CAD build for the part. Positions are in the model's coordinates, mm. A direction names the side the tool comes from. Coordinates: 2 decimals unless noted, no trailing zeros. Order: outer loops, then holes, each group sorted by start corner. A loop starts at its lowest first (then second) coordinate and runs counter-clockwise, first axis right, second up. Notation, with made-up numbers: M 64,48.25 L 70,48.25 A30 ccw 70,83.25 Z; hole C 7,34 d10. An arc over 180 degrees is marked long. Write item = value, one per line.
from build123d import *

# Parameters (mm, degrees)
F1_R     = 1.99999
F2_DEPTH = 25
F6_R     = 2


# Not quite as in the source:
# - a fillet or chamfer that OpenCascade refuses, or shapes differently, is made with other operations: its cross-section is extruded or revolved along the edge and cut away or added
# - a fillet or chamfer is up to 0.001 mm smaller than in the source, because OpenCascade refuses the exact size


with BuildPart() as f0:
    # F3 (on Front) → F0 (revolve)
    with BuildSketch(Plane.XZ):
        Polygon((-2, 0), (0, 0), (0, 12), (-18.8, 12), (-18.8, 13.3), (-20.8, 13.3), (-20.8, 10.2), (-16.5, 10.2), (-15, 10.2), (-11.6, 10.2), (-10.1, 10.2), (-2, 10.2), align=None)
        Polygon((-14.9505181851, 9.7), (-15, 10.2), (-16.5, 10.2), align=None)
        Polygon((-10.2909830056, 9.7), (-10.1, 10.2), (-11.6, 10.2), align=None)
    revolve(axis=Axis((-1, 0, 0), (1, 0, 0)))

    # F1 (radius 2 in the source; OpenCascade refuses exactly that, so slightly less here)
    f1_edges = [f0.edges().sort_by_distance(p)[0] for p in [
        (-20.8, 0, -13.3),
    ]]
    fillet(f1_edges, radius=F1_R)

    # F4: fillet of radius 1.5 on 2 edges, made by hand

    # F4_s1 → F4_t2 (revolve, cut)
    with BuildSketch(Plane.XZ):
        with BuildLine():
            ThreePointArc((-16.1707444356, 10.0937530079), (-15.5745304293, 10.0274099354), (-15, 10.2))
            Line((-15, 10.2), (-14.9505181851, 9.7))
            Line((-14.9505181851, 9.7), (-16.1707444356, 10.0937530079))
        make_face()
    revolve(axis=Axis((-14.9505181851, 0, 0), (1, 0, 0)), mode=Mode.SUBTRACT)

    # F4_s3 → F4_t4 (revolve, cut)
    with BuildSketch(Plane.XZ):
        with BuildLine():
            ThreePointArc((-11.3639501712, 10.1098369884), (-10.721986782, 10.0148974609), (-10.1, 10.2))
            Line((-10.1, 10.2), (-10.2909830056, 9.7))
            Line((-10.2909830056, 9.7), (-11.3639501712, 10.1098369884))
        make_face()
    revolve(axis=Axis((-10.2909830056, 0, 0), (1, 0, 0)), mode=Mode.SUBTRACT)

    # F5 (on Top) → F2 (cut, symmetric)
    with BuildSketch(Plane.XY):
        Polygon((-7.8, 6.5), (-30.9797403524, 6.5), (-30.8855128417, -6.5), (-7.8, -6.5), align=None)
    extrude(amount=F2_DEPTH, both=True, mode=Mode.SUBTRACT)

    # F6
    f6_edges = [f0.edges().sort_by_distance(p)[0] for p in [
        (0, 0, -12),
    ]]
    fillet(f6_edges, radius=F6_R)


solid = f0.part
(1) Tool access for faces 1 (the face through (-18.8, -12.2, -0.8)), 2 (the face through (-16.333, -10.145, 0.125)), 3 (the face through (-13.3, -10.2, 0.1)), 4 (the face through (-18.8, 12.2, 0.1)), 5 (the face through (-7.8, -0.1, -10.4)): list every direction of +Z, -Z, +X, -X, +Y, -Y with a clear straight run to the whole face (end or side of a thin tool).
Evaluation:
face_1 = +X, -Y
face_2 = -X
face_3 = none
face_4 = +X, +Y
face_5 = +Z, -Z, -X
(2) Slice it at A-A, the plane y = 0. Write the cut outline in (x, z).
Evaluation:
outline = M -7.8,-12 L -2,-12 A2 ccw 0,-10 L 0,10 A2 ccw -2,12 L -7.8,12 L -7.8,10.2 L -2,10.2 L -2,-10.2 L -7.8,-10.2 Z
(3) Slice it at B-B, the plane x = -13. Write the cut outline in (y, z).
Evaluation:
outline = M -6.5,-10.09 L -6.5,-7.86 A10.2 cw -6.5,7.86 L -6.5,10.09 A12 ccw Z; M 6.5,-10.09 A12 ccw 6.5,10.09 L 6.5,7.86 A10.2 cw 6.5,-7.86 Z
(4) Pin check, flat tips, straight feed: pin 1 Ø3.5 at (y, z) = (-2, 9) entering from -X; pin 2 Ø2 at (x, z) = (-8.5, 7.5) entering from -Y; pin 3 Ø1 at (y, z) = (1, -8) entering from -X. Stop position of each tip, or through.
Evaluation:
pin_1 = -7.8
pin_2 = -10.09
pin_3 = -2
(5) Wall check: line 1 (Z direction, x = -6.25, y = 0); line 2 (X direction, y = -5.75, z = 2.5). Give the ranges that are in metal, low to high. Write a range as from..to.
Evaluation:
line_1 = -12..-10.2, 10.2..12
line_2 = -2..0
(6) Slice it at D-D, the plane x = -2.75. Write the cut outline in (y, z).
Evaluation:
outline = C 0,0 d24; hole C 0,0 d20.4
(7) Pull direction Z, two halves, no side cores. Call faces 6 (the face through (-10.518, 7.302, -9.523)), 7 (the face through (-18.6, 10.2, -0.1)), 8 (the face through (-20.8, -10.333, 0.642)): +Z half, -Z half, draft (parallel to the pull), parting line (faces both ways), or undercut.
Evaluation:
face_6 = parting line
face_7 = undercut
face_8 = draft
